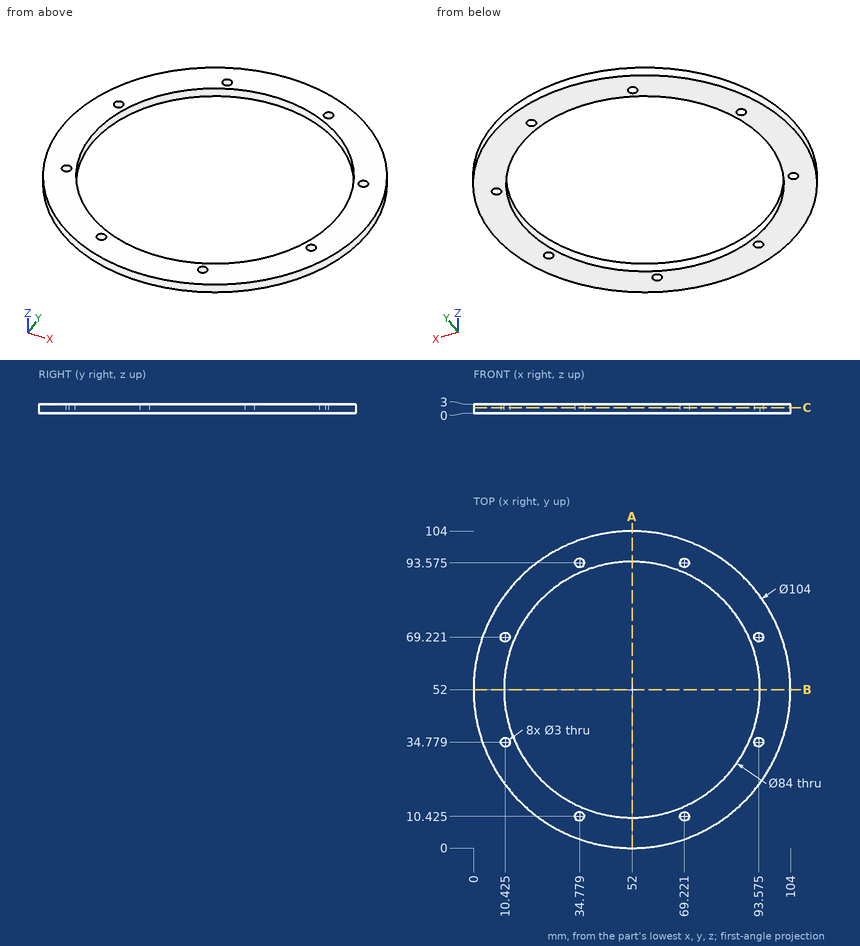
Drawing for the job (mm, zero at the part's lowest x, y, z). Coordinates: 2 decimals unless noted, no trailing zeros. Order: outer loops, then holes, each group sorted by start corner. A loop starts at its lowest first (then second) coordinate and runs counter-clockwise, first axis right, second up.
Item 1: Band-saw the part on A-A on x = 52. List the corners of the cut face in (y, z).
Check sheet entries:
outline: (0, 0) - (10, 0) - (10, 3) - (0, 3) - close; (94, 0) - (104, 0) - (104, 3) - (94, 3) - close
Item 2: Band-saw the part on C-C on z = 1.8. Give the number of separate pieces and of enclosed holes in the cut face, plus the area to 3 significant figures.
Check sheet entries:
separate pieces: 1
enclosed holes: 9
area: 2,900 mm2
Item 3: Pin check, flat tips, straight feed: pin 1 Ø2.5 at (x, y) = (69.22, 10.43) entering from -Z; pin 2 Ø1 at (y, z) = (33.5, 2) entering from -X (1 decimal); pin 3 Ø1 at (y, z) = (74, 2) entering from -X; pin 4 Ø4 at (x, y) = (34.78, 93.57) entering from +Z. Stop position of each tip, or through.
Check sheet entries:
pin 1: passes through
pin 2: stops at x = 3.2
pin 3: stops at x = 4.65
pin 4: stops at z = 3
Item 4: Drill centre lines: L1, parallel to Y at x = 52, z = 1.5; L2, parallel to Y at x = 38, z = 1.2; L3, parallel to X at y = 60.5, z = 1.5. Where is each one in solid material? Low to high.
Check sheet entries:
L1: y = 0 to 10, 94 to 104
L2: y = 1.92 to 12.4, 91.6 to 102.08
L3: x = 0.7 to 10.87, 93.13 to 103.3
